CAD build for the part. Positions are in the model's coordinates, mm. A direction names the side the tool comes from. Round coordinates to 2 decimals unless told otherwise and drop trailing zeros. Write each loop counter-clockwise with the first axis right and the second up, starting at its lowest first coordinate (ties: lowest second). Pieces come first, ordered by that corner, then holes. Notation, with made-up numbers: M 18,-17.5 L 59,-17.5 A22 cw 59,15.5 Z; hole C 35,53.25 d8. An arc over 180 degrees is marked long. Write each question's results on one line, items separated by ' | '. Start each with the question number.
```python
from build123d import *

# Parameters (mm, degrees)
F0_W     = 81.327438
F0_H     = 89.578062
F1_DEPTH = 10
F2_R     = 15.381111
F2_R_2   = 14.786786
F3_DEPTH = 25.4
F4_W     = 76.597116
F4_H     = 81.712402
F5_DEPTH = 5


with BuildPart() as f1:
    # F0 (on Top) → F1 (new body)
    with BuildSketch(Plane.XY):
        Rectangle(F0_W, F0_H)
    extrude(amount=F1_DEPTH)

    # F2 (on face) → F3 (join)
    with BuildSketch(Plane(origin=(0, 0, 0), x_dir=(1, 0, 0), z_dir=(0, 0, -1))):
        with Locations((-20.520471, -20.540299)):
            Circle(F2_R)
        with Locations((22.55322, 21.967739)):
            Circle(F2_R_2)
    extrude(amount=F3_DEPTH)

    # F4 (on face) → F5 (join)
    with BuildSketch(Plane(origin=(0, 0, -25.4), x_dir=(1, 0, 0), z_dir=(0, 0, -1))):
        Rectangle(F4_W, F4_H)
    extrude(amount=F5_DEPTH)


solid = f1.part
```
1) Saw through at C-C, the plane x = -28. Write the cut outline in (y, z).
2) Wall check: line 1 along Z through (x, y) = (-35, 35.5); line 2 along X through (y, z) = (-22, -16.5); line 3 along X through (y, z) = (24, -26.5). Give the ranges that are in metal, low to high. Write a range as from..to.
3) Saw through at A-A, the plane x = 2. Write the cut outline in (y, z), plus the area to 3 significant figures.
4) Saw through at B-B, the plane y = 9. Write the cut outline in (x, z), plus the area to 3 significant figures.
5) Pull direction Z, two halves, no side cores. Call faces 5 (the face through (-1, 1, 0)), 6 (the face through (-1, -1, -30.4)), 7 (the face through (-1, -40.856, -28)): pulls with the +Z half, pulls with the -Z half, needs draft (parallel to the pull), parting line crosses it, or undercut.
6) Drop flat-ended pins along their axis: pin 1 Ø8 at (x, z) = (-10.5, -9.5) entering from -Y; pin 2 Ø12 at (x, z) = (-18.5, -18.5) entering from -Y; pin 3 Ø5.5 at (x, z) = (-13.5, -27) entering from +Y. Give the stop position or say it passes through.
7) Saw through at D-D, the plane z = -6.5. Write the cut outline in (x, y).
8) 3-axis set-ups, long thin cutter, end or side, ignore diameter. For faces 1 (the face through (-1, 40.856, -28)), 2 (the face through (38.299, 1, -28)), 3 (the face through (36.21, -16.3, -12.52)), 4 (the face through (-38.299, 1, -28)): which of +Z, -Z, +X, -X, +Y, -Y reach the whole face in a straight line?
Filled sheet:
1) outline: M -44.79,0 L 7.1,0 L 7.1,-25.4 L -40.86,-25.4 L -40.86,-30.4 L 40.86,-30.4 L 40.86,-25.4 L 33.98,-25.4 L 33.98,0 L 44.79,0 L 44.79,10 L -44.79,10 Z
2) line 1: z = -30.4..-25.4, 0..10 | line 2: x = 7.77..37.34 | line 3: x = -38.3..38.3
3) outline: M -44.79,0 L 44.79,0 L 44.79,10 L -44.79,10 Z; M -40.86,-30.4 L 40.86,-30.4 L 40.86,-25.4 L -40.86,-25.4 Z | area: 1,300 mm^2
4) outline: M -40.66,0 L -30.69,0 L -30.69,-25.4 L -38.3,-25.4 L -38.3,-30.4 L 38.3,-30.4 L 38.3,-25.4 L -10.35,-25.4 L -10.35,0 L 40.66,0 L 40.66,10 L -40.66,10 Z | area: 1,710 mm^2
5) face 5: undercut | face 6: pulls with the -Z half | face 7: needs draft
6) pin 1: stops at y = 6.39 | pin 2: stops at y = 5.16 | pin 3: stops at y = 40.86
7) outline: C -20.52,20.54 d30.76; C 22.55,-21.97 d29.57
8) face 1: -Z, +X, -X, +Y | face 2: -Z, +X, +Y, -Y | face 3: none | face 4: -Z, -X, +Y, -Y
